Model file for the job. Use its own axes, mm. A direction names the side the tool comes from. Coordinates: 2 decimals unless noted, no trailing zeros. Order: outer loops, then holes, each group sorted by start corner. A loop starts at its lowest first (then second) coordinate and runs counter-clockwise, first axis right, second up. Notation, with made-up numbers: M -38.5,14.5 L 17.5,14.5 A19 ccw 17.5,33.5 Z; hole C -13,62.5 d6. An arc over 180 degrees is marked long. Return JSON: item names as keys, results as strings.
```python
from build123d import *

# Parameters (mm, degrees)
PAD_DEPTH   = 12.5
FILLET_R    = 5
FILLET001_R = 8


with BuildPart() as part:
    # Sketch → Pad (new body)
    with BuildSketch(Plane.XY):
        with BuildLine():
            ThreePointArc((-8.5, 2.95804), (0, -9), (8.5, 2.95804))
            ThreePointArc((10.388889, 3.615382), (9.115773, 4.231155), (8.5, 2.95804))
            ThreePointArc((1.5, -10.897247), (9.380326, -5.745387), (10.388889, 3.615382))
            Line((1.5, -30.897247), (1.5, -10.897247))
            Line((-1.5, -30.897247), (1.5, -30.897247))
            Line((-1.5, -10.897247), (-1.5, -30.897247))
            ThreePointArc((-10.388889, 3.615382), (-9.380326, -5.745387), (-1.5, -10.897247))
            ThreePointArc((-8.5, 2.95804), (-9.115773, 4.231155), (-10.388889, 3.615382))
        make_face()
    extrude(amount=PAD_DEPTH)

    # Fillet
    fillet_edges = [part.edges().sort_by_distance(p)[0] for p in [
        (0, -30.897247, 0),
        (0, -30.897247, 12.5),
    ]]
    fillet(fillet_edges, radius=FILLET_R)

    # Fillet001
    fillet001_edges = [part.edges().sort_by_distance(p)[0] for p in [
        (1.5, -10.897247, 6.25),
        (-1.5, -10.897247, 6.25),
    ]]
    fillet(fillet001_edges, radius=FILLET001_R)


solid = part.part
```
Item 1: Drop flat-ended pins along their axis: pin 1 Ø5 at (y, z) = (-9.5, 5.5) entering from -X; pin 2 Ø1 at (x, z) = (4, 4.5) entering from +Y; pin 3 Ø1 at (x, z) = (0, 8.5) entering from +Y. Give the stop position or say it passes through.
Check result:
{"pin 1": "stops at x = -8.49", "pin 2": "stops at y = -7.79", "pin 3": "stops at y = -8.99"}
Item 2: Saw through at C-C (x = 0). Write the cut outline in (y, z).
Check result:
{"outline": "M -30.9,5 A5 ccw -25.9,0 L -9,0 L -9,12.5 L -25.9,12.5 A5 ccw -30.9,7.5 Z"}
Item 3: Saw through at A-A (y = 0). Write the cut outline in (x, z).
Check result:
{"outline": "M -11,0 L -9,0 L -9,12.5 L -11,12.5 Z; M 9,0 L 11,0 L 11,12.5 L 9,12.5 Z"}
Item 4: Wall check: line 1 (X direction, y = 0, z = 7.5); line 2 (X direction, y = -21.5, z = 9.5); line 3 (X direction, y = -3, z = 8). Give the ranges that are in metal, low to high.
Check result:
{"line 1": "x = -11 to -9, 9 to 11", "line 2": "x = -1.5 to 1.5", "line 3": "x = -10.58 to -8.49, 8.49 to 10.58"}
Item 5: 3-axis set-ups, long thin cutter, end or side, ignore diameter. For faces 4 (the flat face through (0, -10, 0)), 5 (the flat face through (-1.5, -24, 6)): which of +Z, -Z, +X, -X, +Y, -Y reach the whole face in a straight line?
Check result:
{"face 4": "-Z, +X, -X, +Y, -Y", "face 5": "+Z, -Z, -X, -Y"}
Item 6: Pull direction Y, two halves, no side cores. Call faces 1 (the cylindrical face through (0.02, -29.47, 11)), 2 (the flat face through (1.5, -24, 6)), 3 (the cylindrical face through (0, -9, 6)): +Y half, -Y half, draft (parallel to the pull), parting line (faces both ways), or undercut.
Check result:
{"face 1": "-Y half", "face 2": "draft", "face 3": "undercut"}
Item 7: Saw through at D-D (z = 10.25). Write the cut outline in (x, y).
Check result:
{"outline": "M -10.39,3.62 A11 ccw -5.5,-9.53 A8 cw -1.5,-16.45 L -1.5,-30.07 L 1.5,-30.07 L 1.5,-16.45 A8 cw 5.5,-9.53 A11 ccw 10.39,3.62 A1 ccw 8.5,2.96 A9 cw long -8.5,2.96 A1 ccw Z"}
Item 8: Saw through at B-B (z = 6). Write the cut outline in (x, y).
Check result:
{"outline": "M -10.39,3.62 A11 ccw -5.5,-9.53 A8 cw -1.5,-16.45 L -1.5,-30.9 L 1.5,-30.9 L 1.5,-16.45 A8 cw 5.5,-9.53 A11 ccw 10.39,3.62 A1 ccw 8.5,2.96 A9 cw long -8.5,2.96 A1 ccw Z"}
